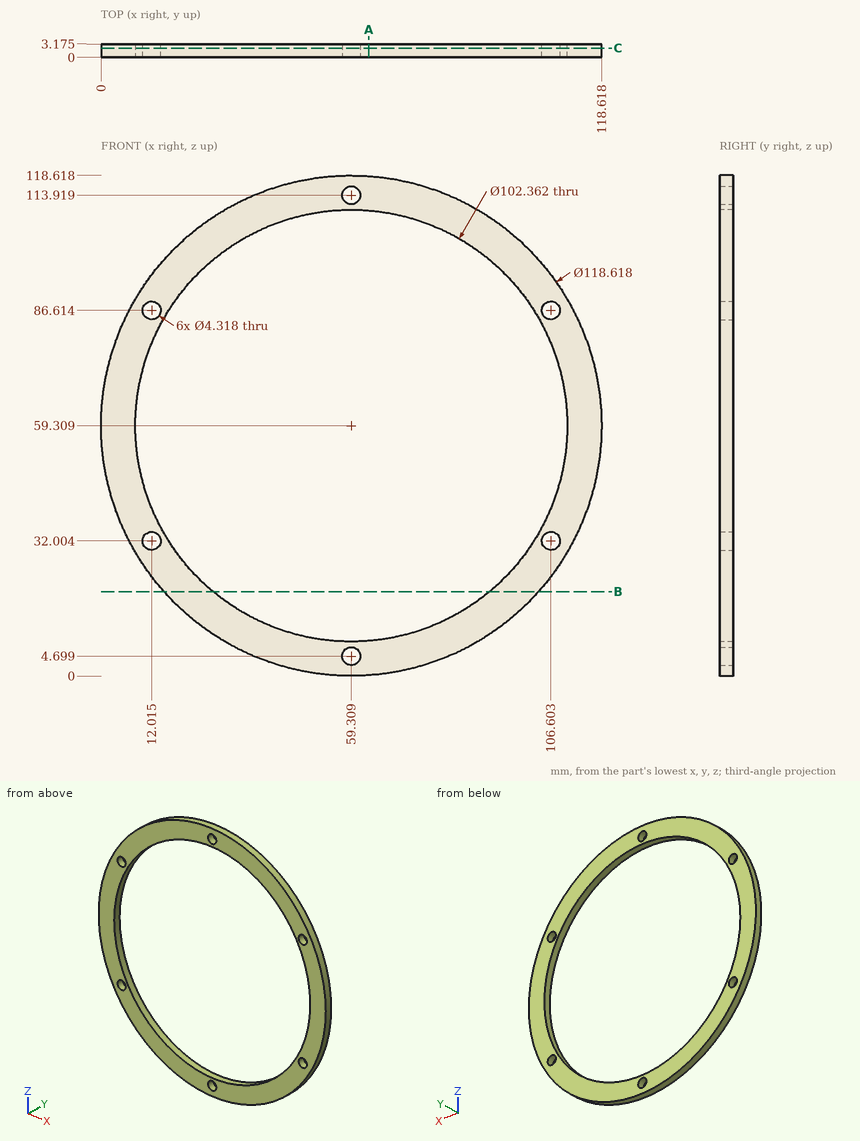
Answer from the drawing. Dimensions are ordinates in mm from the lowest x, y and z of the part. Give positions to 0.01 mm unless a question says otherwise; leave off trailing zeros. Loops run counter-clockwise (first coordinate to the right, second up) from the corner with the lowest first, then second, coordinate; pieces in that order, holes last. Notation, with made-up numbers: (12, 88) -> (18, 88) arc R10 ccw to (18, 95) -> close; hole circle Ø9 at (-15, 4.5). An arc over 180 degrees is marked (long way). Use a Markdown table: item, result.
Q1. Section A-A, the plane x = 63.5 is taken. Determine the outline of the cut face in (y, z) (1 decimal).
Solved:
| item | result |
|---|---|
| outline | (0, 0.1) -> (3.2, 0.1) -> (3.2, 8.3) -> (0, 8.3) -> close; (0, 110.3) -> (3.2, 110.3) -> (3.2, 118.5) -> (0, 118.5) -> close |
Q2. This flat-tipped pin is pushed along its axis until it touches: pin 1 (4 mm diameter, centred on x = 106.6, z = 86.61, fed in from -Y). Where does it stop, or does it pass through?
Solved:
| item | result |
|---|---|
| pin 1 | passes through |
Q3. Find the intervals of material crossed by line 1 along X through (y, z) = (2.15, 87.5) (1 decimal); line 2 along X through (y, z) = (1.05, 40); line 3 along X through (y, z) = (2.7, 6) (1 decimal), in increasing order.
Solved:
| item | result |
|---|---|
| line 1 | x = 7.1 to 10, 14 to 16.6, 102 to 104.6, 108.6 to 111.5 |
| line 2 | x = 3.23 to 11.91, 106.71 to 115.39 |
| line 3 | x = 33.3 to 57.6, 61 to 85.3 |
Q4. Section B-B, the plane z = 20 is taken. Determine the outline of the cut face in (x, y) (1 decimal).
Solved:
| item | result |
|---|---|
| outline | (14.9, 0) -> (26.5, 0) -> (26.5, 3.2) -> (14.9, 3.2) -> close; (92.1, 0) -> (103.7, 0) -> (103.7, 3.2) -> (92.1, 3.2) -> close |
Q5. Section C-C, the plane y = 2.2 is taken. Count the separate pieces of the cut face and the enclosed holes in it, then the cut area to 3 significant figures.
Solved:
| item | result |
|---|---|
| separate pieces | 1 |
| enclosed holes | 7 |
| area | 2,730 mm^2 |
